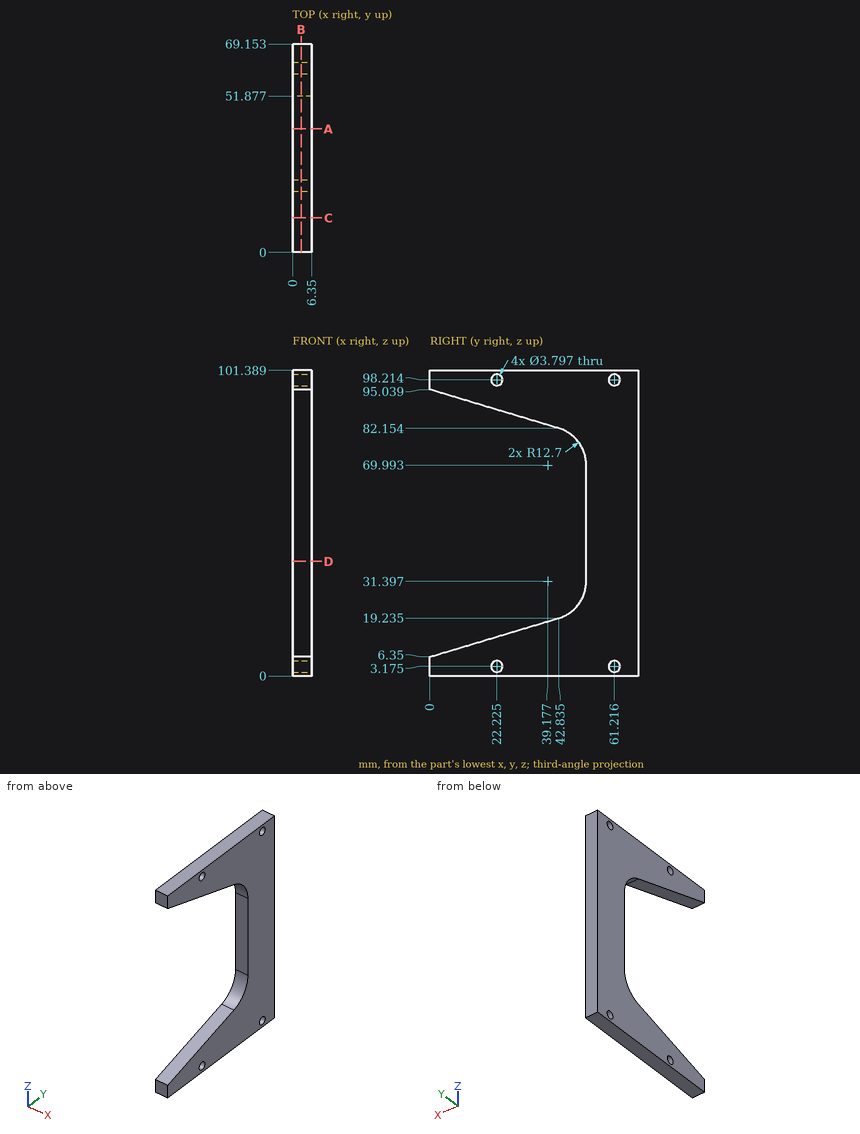
Geometry check sheet. Reference: drawing and pictorial views, mm from the part's lowest x, y, z. Round coordinates to 2 decimals unless told otherwise and drop trailing zeros. Order: outer loops, then holes, each group sorted by start corner. A loop starts at its lowest first (then second) coordinate and runs counter-clockwise, first axis right, second up. Notation, with made-up numbers: (50.25, -5.75) - (66.25, -5.75) arc R7 cw to (66.25, 4.25) - close; hole circle Ø10 at (82, 82). An arc over 180 degrees is marked (long way). Write item = value, one per line.
Q1. Go/stop test with flat-tipped pins: pin 1 (1.9 mm diameter, centred on x = 3, z = 54.5, fed in from -Y); pin 2 (1.5 mm diameter, centred on y = 60, z = 56, fed in from -X); pin 3 (3 mm diameter, centred on x = 3.5, z = 76, fed in from -Y). Record where each tip stops, or that it passes through.
Computed:
pin_1 = 51.88
pin_2 = 0
pin_3 = 49.42
Q2. Section check A-A (y = 41). Record the boundary of the cut face in (x, z).
Computed:
outline = (0, 0) - (6.35, 0) - (6.35, 18.68) - (0, 18.68) - close; (0, 82.71) - (6.35, 82.71) - (6.35, 101.39) - (0, 101.39) - close
Q3. Thickness scan on line 1 along Z through (x, y) = (0.75, 59.5) (1 decimal); line 2 along Y through (x, z) = (0.75, 45.5); line 3 along Z through (x, y) = (4, 38). Record the ranges inside material, lowest first.
Computed:
line_1 = 0 to 2.4, 4 to 97.4, 99 to 101.4
line_2 = 51.88 to 69.15
line_3 = 0 to 17.78, 83.61 to 101.39
Q4. Section check C-C (y = 11.5). Record the boundary of the cut face in (x, z), and give its area (3 significant figures).
Computed:
outline = (0, 0) - (6.35, 0) - (6.35, 9.81) - (0, 9.81) - close; (0, 91.58) - (6.35, 91.58) - (6.35, 101.39) - (0, 101.39) - close
area = 125 mm^2
Q5. Section check B-B (x = 2.75). State how many separate pieces and enclosed holes the cut face has, and give its area (3 significant figures).
Computed:
separate_pieces = 1
enclosed_holes = 4
area = 3,210 mm^2
Q6. Section check D-D (z = 38). Record the boundary of the cut face in (x, y), and give its area (3 significant figures).
Computed:
outline = (0, 51.88) - (6.35, 51.88) - (6.35, 69.15) - (0, 69.15) - close
area = 110 mm^2
